Autodesk Inventor part; units mm, degrees
ref_plane "YZ Plane" through (0, 0, 0) normal (1, 0, 0) x (0, 1, 0)
ref_plane "XZ Plane" through (0, 0, 0) normal (0, 1, 0) x (-1, 0, 0)
ref_plane "XY Plane" through (0, 0, 0) normal (0, 0, 1) x (1, 0, 0)
sketch "Sketch1" plane through (0, 0, 0) normal (0, 1, 0) x (-1, 0, 0)
  circle A0 centre (0, 0) radius 37.5
  dimension "d0" = 75
extrude "Extrusion1" add sketch "Sketch1" along normal blind 30
sketch "Sketch6" plane through (0, 30, 0) normal (0, 1, 0) x (1, 0, 0)
  circle A0 centre (0, 0) radius 30
  circle A1 centre (0, 0) radius 25
  circle A2 centre (0, 0) radius 7.5
  dimension "d16" = 60
  dimension "d17" = 50
  dimension "d28" = 15
extrude "Extrusion5" add sketch "Sketch6" along normal blind 10 contours A0
sketch "Sketch9" plane through (0, 0, 0) normal (0, 0, 1) x (1, 0, 0)
  line L0 (0, 0) -> (30, 0)
  line L1 (30, 0) -> (30, -40)
  line L2 (30, -40) -> (0, -40)
  line L3 (0, -40) -> (0, 0)
  circle A0 centre (0, -40) radius 30
  line L4 (-30, 0) -> (-30, -40)
  line L5 (0, 0) -> (-30, 0)
  line L6 (37.5, 30) -> (-37.5, 30)
  point P0 (-30, -40)
  point P1 (30, -40)
  dimension "d38" = 40
  dimension "d40" = 60
  dimension "d41" = 30
  dimension "d44" = 0
extrude "Extrusion8" add sketch "Sketch9" along normal blind 22
properties part number "Shoulder1"
Geometry: final body of the model. Coordinates: model frame, mm. A direction names the side the tool comes from. Round coordinates to 2 decimals unless told otherwise and drop trailing zeros. Write each loop counter-clockwise with the first axis right and the second up, starting at its lowest first coordinate (ties: lowest second). Pieces come first, ordered by that corner, then holes.
Item 1: Pin query (flat end, axial travel): P1, Ø1.5, axis at x = 15.5, y = -37, coming from the -Z side; P2, Ø8, axis at x = -18, y = 24, coming from the -Z side; P3, Ø4, axis at x = -0.5, z = 27.5, coming from the -Y side. Return the tip coordinate at first contact, or that it passes through.
Item 2: Section query C-C (y = -23.5). Return loops of the section in (x, z), plus the area to 3 significant figures.
Item 3: Section query B-B (z = 1.5). Return loops of the section in (x, y), plus the area to 3 significant figures.
Item 4: Section query A-A (x = 0). Return loops of the section in (y, z).
Item 5: Set-up query: faces 4 (the face through (0, -35, 0)), 5 (the face through (0, -35, 22)), 6 (the face through (17, 30, 25)), 7 (the face through (-30, -20, 11)). Return all of +Z, -Z, +X, -X, +Y, -Y with unobstructed straight access to the full face (end or side cutting, diameter ignored); none if empty.
Item 6: Mould query, pull axis Z, two halves, no side actions, for faces 1 (the face through (0, 30, 0)), 2 (the face through (4.88, 14.79, -37.18)), 3 (the face through (30, -20, 11)). Classes: +Z half, -Z half, draft (parallel to the pull), parting line (faces both ways), or undercut.
Item 7: Material intervals for L1, parallel to X at y = 38, z = 0; L2, parallel to Z at x = 6, y = -19, sorted ascending.
Item 8: Section query D-D (z = -11). Return loops of the section in (x, y).
Completed:
1. P1: stops at z = 0
1. P2: stops at z = -34.79
1. P3: stops at y = 0
2. outline: (-30, 0) - (30, 0) - (30, 22) - (-30, 22) - close
2. area: 1,320 mm2
3. outline: (-37.47, 0) - (-30, 0) - (-30, -40) arc R30 ccw to (30, -40) - (30, 0) - (37.47, 0) - (37.47, 30) - (29.96, 30) - (29.96, 40) - (24.95, 40) - (24.95, 30) - (-24.95, 30) - (-24.95, 40) - (-29.96, 40) - (-29.96, 30) - (-37.47, 30) - close
3. area: 6,160 mm2
4. outline: (-70, 0) - (0, 0) - (0, -37.5) - (30, -37.5) - (30, -30) - (40, -30) - (40, -25) - (30, -25) - (30, 25) - (40, 25) - (40, 30) - (30, 30) - (30, 37.5) - (0, 37.5) - (0, 22) - (-70, 22) - close
5. face 4: -Z, +X, -X, -Y
5. face 5: +Z, +X, -X, -Y
5. face 6: +Y
5. face 7: +Z, -Z, -X, -Y
6. face 1: undercut
6. face 2: parting line
6. face 3: draft
7. L1: x = -30 to -25, 25 to 30
7. L2: z = 0 to 22
8. outline: (-35.85, 0) - (35.85, 0) - (35.85, 30) - (27.91, 30) - (27.91, 40) - (22.45, 40) - (22.45, 30) - (-22.45, 30) - (-22.45, 40) - (-27.91, 40) - (-27.91, 30) - (-35.85, 30) - close
